Work out the finished part from the listing and answer in its coordinate system (mm). Face numbers are marked on the shaded views. A direction names the side the tool comes from. Round coordinates to 2 decimals unless told otherwise and drop trailing zeros. Order: outer loops, then holes, each group sorted by start corner. A loop starts at its lowest first (then second) coordinate and runs counter-clockwise, first axis right, second up. Notation, with made-up numbers: (-10.75, 24) - (31.25, 24) arc R19 cw to (31.25, 33) - close; hole circle Ø4 at (72.25, 40.5). An arc over 180 degrees is marked (long way). Answer in a Markdown table with one row per item.
from build123d import *

# Parameters (mm, degrees)
SKETCH1_R           = 15
SKETCH1_R_2         = 1.5
SKETCH1_R_3         = 5
BOSS_EXTRUDE1_DEPTH = 2
SKETCH1_3_R         = 5
SKETCH1_3_R_2       = 3.5
SKETCH1_3_R_3       = 3.2
BOSS_EXTRUDE2_DEPTH = 17
BOSS_EXTRUDE3_START = 17
SKETCH1_4_R         = 3.5
SKETCH1_4_R_2       = 3.2
BOSS_EXTRUDE3_DEPTH = 16
SKETCH2_R           = 3.2
BOSS_EXTRUDE4_DEPTH = 13
FILLET1_R           = 1


with BuildPart() as part:
    # Sketch1 → Boss-Extrude1 (new body)
    with BuildSketch(Plane.XY):
        Circle(SKETCH1_R)
        with Locations((0, 12.5)):
            Circle(SKETCH1_R_2, mode=Mode.SUBTRACT)
        with Locations((12.5, 0)):
            Circle(SKETCH1_R_2, mode=Mode.SUBTRACT)
        with Locations((0, -12.5)):
            Circle(SKETCH1_R_2, mode=Mode.SUBTRACT)
        with Locations((-12.5, 0)):
            Circle(SKETCH1_R_2, mode=Mode.SUBTRACT)
        Circle(SKETCH1_R_3, mode=Mode.SUBTRACT)
    extrude(amount=BOSS_EXTRUDE1_DEPTH)

    # Sketch1<3> → Boss-Extrude2 (add)
    # profile 1 of 3: a face of its own
    with BuildSketch(Plane.XY):
        Circle(SKETCH1_3_R)
        Circle(SKETCH1_3_R_2, mode=Mode.SUBTRACT)
    # profile 2 of 3: a face of its own
    with BuildSketch(Plane.XY):
        Circle(SKETCH1_3_R_2)
        Circle(SKETCH1_3_R_3, mode=Mode.SUBTRACT)
    # profile 3 of 3: a face of its own
    with BuildSketch(Plane.XY):
        Circle(SKETCH1_3_R_3)
    extrude(amount=BOSS_EXTRUDE2_DEPTH)

    # Sketch1<4> → Boss-Extrude3 (add)
    with BuildSketch(Plane.XY.offset(BOSS_EXTRUDE3_START)):
        Circle(SKETCH1_4_R)
        Circle(SKETCH1_4_R_2, mode=Mode.SUBTRACT)
    extrude(amount=BOSS_EXTRUDE3_DEPTH)

    # Sketch2 → Boss-Extrude4 (add)
    with BuildSketch(Plane.XY.offset(17)):
        Circle(SKETCH2_R)
    extrude(amount=BOSS_EXTRUDE4_DEPTH)

    # Fillet1
    fillet1_edges = [part.edges().sort_by_distance(p)[0] for p in [
        (-3.5, 0, 17),
    ]]
    fillet(fillet1_edges, radius=FILLET1_R)


solid = part.part
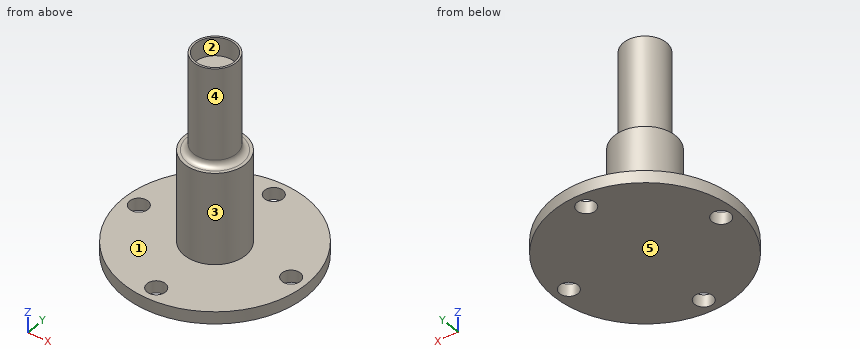
1) The mould has two halves that part along X. Classify the marked faces 1, 2 and 3: released by +X, released by -X, zero draft, split by the parting line, or undercut.
Filled in:
| item | result |
|---|---|
| face 1 | zero draft |
| face 2 | undercut |
| face 3 | split by the parting line |
2) Which of the six approach directions +Z, -Z, +X, -X, +Y, -Y give full straight-line access (tool end or side, diameter ignored) to the marked faces 4 and 5?
Filled in:
| item | result |
|---|---|
| face 4 | +Z |
| face 5 | -Z, +X, -X, +Y, -Y |
3) Each of these flat-tipped pins is pushed along its axis until it touches: pin 1 (2.5 mm diameter, centred on x = 0, y = -12.5, fed in from +Z); pin 2 (3 mm diameter, centred on x = -2.5, z = 21, fed in from -Y); pin 3 (1.5 mm diameter, centred on x = -6.5, y = 6, fed in from +Z); pin 4 (10 mm diameter, centred on y = 8.5, z = 4, fed in from -X). Where does it stop, or does it pass through?
Filled in:
| item | result |
|---|---|
| pin 1 | passes through |
| pin 2 | stops at y = -3.35 |
| pin 3 | stops at z = 2 |
| pin 4 | stops at x = -14.48 |
4) Find the intervals of material crossed by probe 1 along Y at (x, z) = (0, 1.25); probe 2 along Y at (x, z) = (0, 31.15); probe 3 along Z at (x, y) = (2.25, 9.75), in increasing order. Write a range as from..to.
Filled in:
| item | result |
|---|---|
| probe 1 | y = -15..-14, -11..11, 14..15 |
| probe 2 | y = -3.5..-3.2, 3.2..3.5 |
| probe 3 | z = 0..2 |
5) Find section C-C, the plane y = 12.5. Give the vertices of the cut face in (x, z).
Filled in:
| item | result |
|---|---|
| outline | (-8.29, 0) - (-1.5, 0) - (-1.5, 2) - (-8.29, 2) - close; (1.5, 0) - (8.29, 0) - (8.29, 2) - (1.5, 2) - close |
6) Find section A-A, the plane y = 0. Give the vertices of the cut face in (x, z).
Filled in:
| item | result |
|---|---|
| outline | (-15, 0) - (-14, 0) - (-14, 2) - (-15, 2) - close; (-11, 0) - (11, 0) - (11, 2) - (5, 2) - (5, 17) - (4.5, 17) arc R1 cw to (3.5, 18) - (3.5, 33) - (3.2, 33) - (3.2, 30) - (-3.2, 30) - (-3.2, 33) - (-3.5, 33) - (-3.5, 18) arc R1 cw to (-4.5, 17) - (-5, 17) - (-5, 2) - (-11, 2) - close; (14, 0) - (15, 0) - (15, 2) - (14, 2) - close |
